Here's how the part is built. I have some questions about the finished solid (model axes, mm). A direction names the side the tool comes from. Give positions to 0.01 mm unless a question says otherwise; leave off trailing zeros. Write each loop counter-clockwise with the first axis right and the second up, starting at its lowest first coordinate (ties: lowest second). Pieces come first, ordered by that corner, then holes. Notation, with made-up numbers: (-12, 62.25) - (30, 62.25) arc R13 cw to (30, 73.25) - close; hole circle Ø2 at (41, 46.25). An arc over 180 degrees is marked (long way). One line per item, written item: value. Start each with the question number.
1) We'd pull the mould along Z, two halves only. Please class faces 6 (the cylindrical face through (0, -11, -1)), 7 (the flat face through (0, -9, -2)), 8 (the flat face through (4, -19, 10)), 9 (the flat face through (19, -22, 0.9)): +Z half, -Z half, draft (parallel to the pull), parting line (faces both ways), or undercut.
2) Imagine slicing it at C-C on y = -12.75. Write out the boundary of the cut face in (x, z).
3) Imagine slicing it at A-A on z = 4. Count the separate pieces of the cut face and the enclosed holes in it, plus the area to 3 significant figures.
4) I'm going to push flat-ended pins straight in: P1, Ø1.8, axis at x = -9.5, z = 4, coming from the -Y side; P2, Ø1, axis at y = -8.5, z = 6.5, coming from the -X side; P3, Ø3, axis at x = 16.5, z = 4, coming from the -Y side; P4, Ø2, axis at y = -20.5, z = -1.5, coming from the -X side. Where does each tip first touch, or does it pass through?
5) Please list where these lines run through material, in increasing order: L1, parallel to Y at x = 0, z = -1.25; L2, parallel to Z at x = 18, y = -20.25; L3, parallel to X at y = -0.5, z = -1. Write a range as [from, to].
6) Imagine slicing it at B-B on x = 0. Write out the boundary of the cut face in (y, z), plus the area to 3 significant figures.
7) Imagine slicing it at D-D on y = -21.5. Write out the boundary of the cut face in (x, z).
8) On a 3-axis mill with a long thin cutter (end or side, diameter ignored), from which of +Z, -Z, +X, -X, +Y, -Y can I reach the whole of each face in a straight line? I mean faces 1 (the flat face through (-11, -22, 0.9)), 2 (the flat face through (0, -8, 0)), 3 (the cylindrical face through (14.9, -22.4, 4.1)), 4 (the cylindrical face through (-11.081, 0.526, -1.014)), 5 (the flat face through (18, -20, 4)). Say none if no direction works.
from build123d import *
from build123d.topology import SkipClean

# Parameters (mm, degrees)
CROQUIS1_R              = 18
SALIENTE_EXTRUIR1_DEPTH = 10
SALIENTE_EXTRUIR2_START = -12
CROQUIS2_R              = 7
CROQUIS2_R_2            = 1.75
SALIENTE_EXTRUIR2_DEPTH = 2
CROQUIS7_R              = 1.75
CORTAR_EXTRUIR3_DEPTH   = 8
CORTAR_EXTRUIR4_DEPTH   = 3.2


with BuildPart() as part:
    # Croquis1 → Saliente-Extruir1 (new body)
    with BuildSketch(Plane.XY):
        with BuildLine():
            Line((-13, -28), (21, -28))
            Line((21, -28), (21, 0))
            ThreePointArc((21, 0), (-9.16515139, 18.894443628), (-13, -16.492422502))
            Line((-13, -16.492422502), (-13, -28))
        make_face()
        Circle(CROQUIS1_R, mode=Mode.SUBTRACT)
    extrude(amount=SALIENTE_EXTRUIR1_DEPTH)

    # Croquis2 → Saliente-Extruir2 (add)
    with SkipClean():  # the faces are left unmerged after this step: merging them gives an invalid solid
        with BuildSketch(Plane.XY.offset(10).offset(SALIENTE_EXTRUIR2_START)):
            with BuildLine():
                Line((21, 0), (21, -28))
                Line((21, -28), (-13, -28))
                Line((-13, -28), (-13, -16.492422502))
                ThreePointArc((-13, -16.492422502), (-9.16515139, 18.894443628), (21, 0))
            make_face()
            Circle(CROQUIS2_R, mode=Mode.SUBTRACT)
            with Locations((0, -12.75)):
                Circle(CROQUIS2_R_2, mode=Mode.SUBTRACT)
            with Locations((0, 12.75)):
                Circle(CROQUIS2_R_2, mode=Mode.SUBTRACT)
            with Locations((-12.75, 0)):
                Circle(CROQUIS2_R_2, mode=Mode.SUBTRACT)
        extrude(amount=SALIENTE_EXTRUIR2_DEPTH)

    # Croquis7 → Cortar-Extruir3 (cut)
    with SkipClean():  # the faces are left unmerged after this step: merging them gives an invalid solid
        with BuildSketch(Plane.XZ.offset(28)):
            with Locations((-10, 4)):
                Circle(CROQUIS7_R)
            with Locations((18, 4)):
                Circle(CROQUIS7_R)
        extrude(amount=-CORTAR_EXTRUIR3_DEPTH, mode=Mode.SUBTRACT)

    # Croquis8 → Cortar-Extruir4 (cut)
    with SkipClean():  # the faces are left unmerged after this step: merging them gives an invalid solid
        with BuildSketch(Plane(origin=(0, -24, 0), x_dir=(-1, 0, 0), z_dir=(0, -1, 0))):
            with BuildLine():
                Line((-18, -0.9), (-21, -0.9))
                Line((-21, -0.9), (-21, -7.1))
                Line((-21, -7.1), (-18, -7.1))
                ThreePointArc((-18, -7.1), (-14.9, -4), (-18, -0.9))
            make_face()
            with BuildLine():
                Line((10, -0.9), (13, -0.9))
                Line((13, -0.9), (13, -7.1))
                Line((13, -7.1), (10, -7.1))
                ThreePointArc((10, -7.1), (6.9, -4), (10, -0.9))
            make_face()
        extrude(amount=-CORTAR_EXTRUIR4_DEPTH, mode=Mode.SUBTRACT)


solid = part.part
Numbers:
1. face 6: draft
1. face 7: -Z half
1. face 8: +Z half
1. face 9: undercut
2. outline: (-16.69, -2) - (-1.75, -2) - (-1.75, 0) - (-12.71, 0) - (-12.71, 10) - (-16.69, 10) - close; (1.75, -2) - (21, -2) - (21, 10) - (12.71, 10) - (12.71, 0) - (1.75, 0) - close
3. separate pieces: 3
3. enclosed holes: 1
3. area: 646 mm^2
4. P1: y = -20
4. P2: x = -19.42
4. P3: y = -28
4. P4: x = -13
5. L1: [-28, -14.5], [-11, -7], [7, 11], [14.5, 21]
5. L2: [-2, 2.25], [5.75, 10]
5. L3: [-20.99, -14.43], [-11.07, -6.98], [6.98, 21]
6. outline: (-28, -2) - (-14.5, -2) - (-14.5, 0) - (-18, 0) - (-18, 10) - (-28, 10) - close; (-11, -2) - (-7, -2) - (-7, 0) - (-11, 0) - close; (7, -2) - (11, -2) - (11, 0) - (7, 0) - close; (14.5, -2) - (21, -2) - (21, 10) - (18, 10) - (18, 0) - (14.5, 0) - close
6. area: 186 mm^2
7. outline: (-13, -2) - (21, -2) - (21, 0.9) - (18, 0.9) arc R3.1 cw to (18, 7.1) - (21, 7.1) - (21, 10) - (-13, 10) - (-13, 7.1) - (-10, 7.1) arc R3.1 cw to (-10, 0.9) - (-13, 0.9) - close
8. face 1: -X
8. face 2: +Z
8. face 3: +X
8. face 4: +Z, -Z
8. face 5: -Y
